Answer from the drawing. Dimensions are ordinates in mm from the lowest x, y and z of the part. A direction names the side the tool comes from. Give positions to 0.01 mm unless a question says otherwise; leave off trailing zeros. Loops run counter-clockwise (first coordinate to the right, second up) from the corner with the lowest first, then second, coordinate; pieces in that order, holes last.
Item 1: A tool of negligible diameter and unlimited length cuts with its end or side. For the marked faces 4 and 5, from which of +Z, -Z, +X, -X, +Y, -Y can it reach the whole face along a straight path? Write none if from no direction.
Item 2: Section C-C, the plane y = 30.5 is taken. Give the vertices of the cut face in (x, z).
Item 3: Section D-D, the plane y = 15 is taken. Give the vertices of the cut face in (x, z), and give its area (3 significant figures).
Item 4: Each of these flat-tipped pins is pushed along its axis until it touches: pin 1 Ø3 at (x, z) = (21, 9) entering from +Y; pin 2 Ø3 at (x, z) = (19, 19) entering from +Y; pin 3 Ø12 at (x, y) = (20.5, 18.5) entering from -Z. Where does it stop, or does it pass through?
Item 5: The mould has two halves that part along X. Classify the marked faces 1, 2 and 3: pulls with the +X half, pulls with the -X half, needs draft (parallel to the pull), parting line crosses it, or undercut.
Item 6: Consider line 1 along X through (y, z) = (8, 19); line 2 along Z through (x, y) = (19, 29); line 3 along Y through (x, z) = (14, 27). Determine where each line is inside the solid, lowest interval first.
Item 7: Section B-B, the plane z = 19 is taken. Give the vertices of the cut face in (x, y).
Item 8: Section A-A, the plane x = 19 is taken. Give the vertices of the cut face in (y, z), and give its area (3 significant figures).
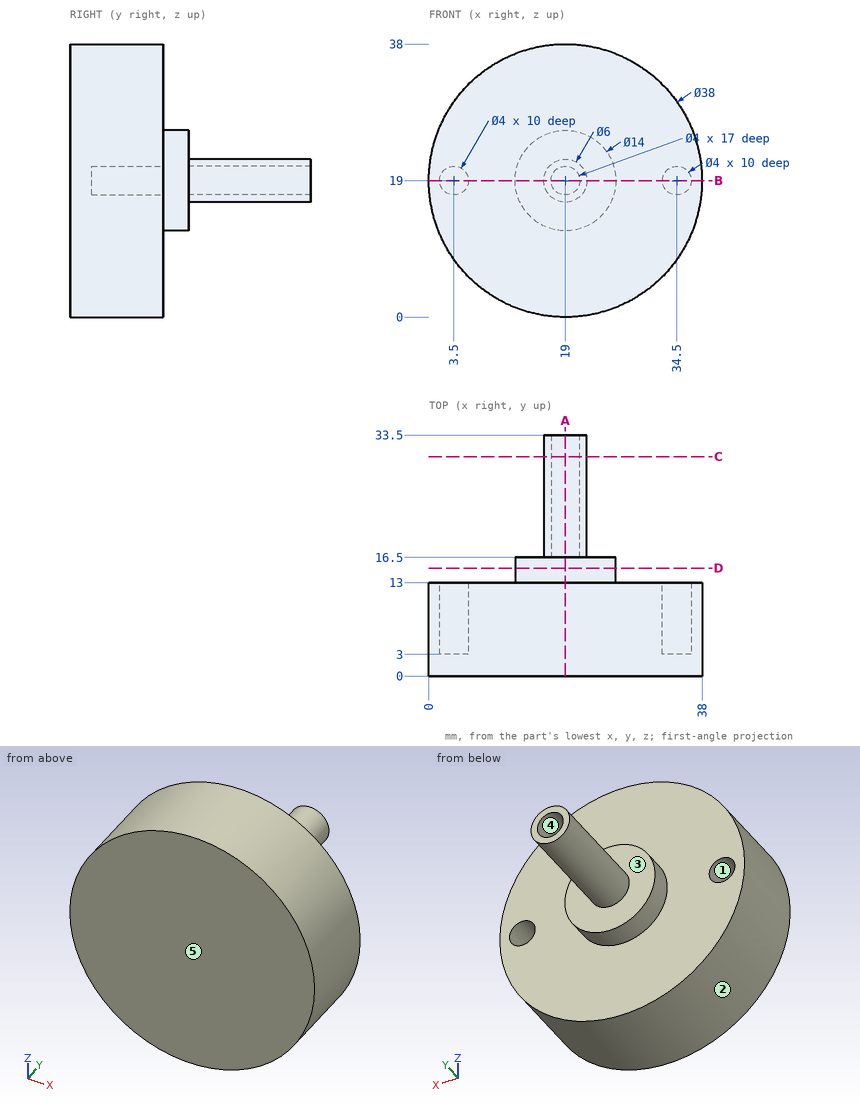
Worked answers:
1. face 4: +Y
1. face 5: +Z, -Z, +X, -X, -Y
2. outline: circle Ø6 at (19, 19); hole circle Ø4 at (19, 19)
3. outline: circle Ø14 at (19, 19)
3. area: 154 mm2
4. pin 1: stops at y = 13
4. pin 2: stops at y = 16.5
4. pin 3: stops at z = 0
5. face 1: undercut
5. face 2: parting line crosses it
5. face 3: needs draft
6. line 1: x = 0 to 1.5, 5.5 to 32.5, 36.5 to 38
6. line 2: z = 16 to 17, 21 to 22
6. line 3: y = 0 to 13
7. outline: (0, 0) - (38, 0) - (38, 13) - (36.5, 13) - (36.5, 3) - (32.5, 3) - (32.5, 13) - (26, 13) - (26, 16.5) - (22, 16.5) - (22, 33.5) - (21, 33.5) - (21, 16.5) - (17, 16.5) - (17, 33.5) - (16, 33.5) - (16, 16.5) - (12, 16.5) - (12, 13) - (5.5, 13) - (5.5, 3) - (1.5, 3) - (1.5, 13) - (0, 13) - close
8. outline: (0, 0) - (13, 0) - (13, 12) - (16.5, 12) - (16.5, 16) - (33.5, 16) - (33.5, 17) - (16.5, 17) - (16.5, 21) - (33.5, 21) - (33.5, 22) - (16.5, 22) - (16.5, 26) - (13, 26) - (13, 38) - (0, 38) - close
8. area: 577 mm2
